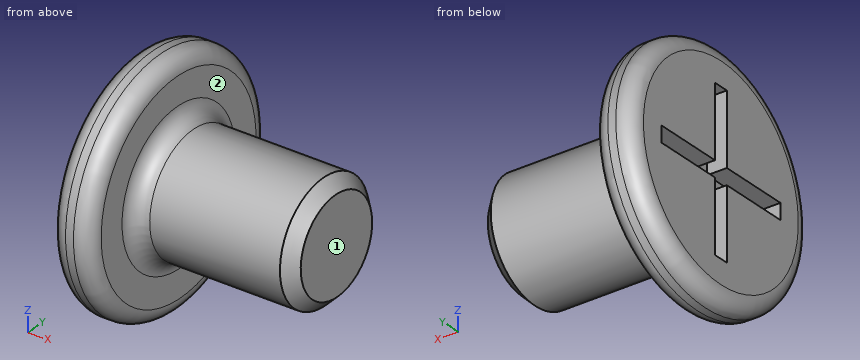
from build123d import *

# Parameters (mm, degrees)
FILLET_1_R          = 0.4
CUT_EXTRUDE_1_DEPTH = 0.5
CHAMFER_1_SIZE      = 0.3


with BuildPart() as part:
    # Эскиз1 → Повернуть1 (revolve)
    with BuildSketch(Plane.XY, mode=Mode.PRIVATE) as revolve_1_sk:
        Polygon((0, 0), (0, 3), (1, 3), (1, 1.5), (5, 1.5), (5, 0), align=None)
    revolve(revolve_1_sk.sketch.rotate(Axis((-40.588436676, 0, 0), (1, 0, 0)), 90), axis=Axis((-40.588436676, 0, 0), (1, 0, 0)))

    # Скругление1
    fillet_1_edges = [part.edges().sort_by_distance(p)[0] for p in [
        (1, 0, -1.5),
        (1, 0, -3),
        (0, 0, -3),
    ]]
    fillet(fillet_1_edges, radius=FILLET_1_R)

    # Эскиз2 → Вырез-Вытянуть1 (cut)
    with BuildSketch(Plane.ZY):
        Polygon((0.2, -2), (-0.2, -2), (-0.2, -0.2), (-2, -0.2), (-2, 0.2), (-0.2, 0.2), (-0.2, 2), (0.2, 2), (0.2, 0.2), (2, 0.2), (2, -0.2), (0.2, -0.2), align=None)
    extrude(amount=-CUT_EXTRUDE_1_DEPTH, mode=Mode.SUBTRACT)

    # Фаска1
    chamfer_1_edges = [part.edges().sort_by_distance(p)[0] for p in [
        (5, 0, -1.5),
    ]]
    chamfer(chamfer_1_edges, length=CHAMFER_1_SIZE)


solid = part.part
Read the model definition and answer for the solid it produces. Units are mm, in the model's axes. Face numbers are marked on the shaded views. A direction names the side the tool comes from. Give positions to 0.01 mm unless a question says otherwise; leave off trailing zeros. Write each loop counter-clockwise with the first axis right and the second up, starting at its lowest first coordinate (ties: lowest second). Pieces come first, ordered by that corner, then holes. Notation, with made-up numbers: M 45.25,60 L 57.25,60 A9 ccw 57.25,64 Z; hole C 86,-30 d3. An arc over 180 degrees is marked long. One line per item, written item: value. Start each with the question number.
(1) Find the intervals of material crossed by line 1 (Z direction, x = 2.15, y = 0.05); line 2 (Y direction, x = 0.4, z = -1.75); line 3 (X direction, y = -2.1, z = -1.2), in increasing order.
(2) Find section B-B (z = 0). Determine the outline of the cut face in (x, y), plus the area to 3 significant figures.
(3) A flat-ended cylindrical pin translates along its axis: pin 1 Ø2 at (y, z) = (0.5, 0.5) entering from -X. Find the tip coordinate at first contact, or state that the pin passes through.
(4) Find section D-D (x = 3.05). Determine the outline of the cut face in (y, z), plus the area to 3 significant figures.
(5) A tool of negligible diameter and unlimited length cuts with its end or side. For the marked faces 1 and 2, from which of +Z, -Z, +X, -X, +Y, -Y can it reach the whole face along a straight path? Write none if from no direction.
(6) Find section A-A (x = 0.3). Determine the outline of the cut face in (y, z), plus the area to 3 significant figures.
Results below:
1. line 1: z = -1.5 to 1.5
1. line 2: y = -2.44 to -0.2, 0.2 to 2.44
1. line 3: x = 0 to 1
2. outline: M 0,-2.6 A0.4 ccw 0.4,-3 L 0.6,-3 A0.4 ccw 1,-2.6 L 1,-1.9 A0.4 cw 1.4,-1.5 L 4.7,-1.5 L 5,-1.2 L 5,1.2 L 4.7,1.5 L 1.4,1.5 A0.4 cw 1,1.9 L 1,2.6 A0.4 ccw 0.6,3 L 0.4,3 A0.4 ccw 0,2.6 L 0,2 L 0.5,2 L 0.5,-2 L 0,-2 Z
2. area: 15.8 mm^2
3. pin 1: stops at x = 0
4. outline: C 0,0 d3
4. area: 7.07 mm^2
5. face 1: +Z, -Z, +X, +Y, -Y
5. face 2: +X
6. outline: C 0,0 d5.97; hole M -2,-0.2 L -0.2,-0.2 L -0.2,-2 L 0.2,-2 L 0.2,-0.2 L 2,-0.2 L 2,0.2 L 0.2,0.2 L 0.2,2 L -0.2,2 L -0.2,0.2 L -2,0.2 Z
6. area: 25.0 mm^2
